Could you check a few things on this model? Use its own coordinates, in mm. A direction names the side the tool comes from. Give positions to 0.01 mm unless a question says otherwise; leave off trailing zeros. Order: outer loops, then holes, each group sorted by start corner. A loop starts at its lowest first (then second) coordinate and runs counter-clockwise, first axis right, second up. Notation, with made-up numbers: M 74.25,63 L 96.25,63 A21 cw 96.25,81 Z; hole C 72.25,51 d7. An arc over 180 degrees is marked long. Use a Markdown table: item, result. Add a question column.
Item 1: I'm going to push flat-ended pins straight in: pin 1 Ø1.2 at (x, y) = (-14, -3) entering from +Z; pin 2 Ø4.5 at (y, z) = (-2.5, 44) entering from -X; pin 3 Ø4 at (x, y) = (-9.5, 0) entering from +Z. Where does each tip first touch, or does it pass through?
Item 2: If we mould it in two halves opening along X, with no side actions, what happens to faces 4 (the face through (26.682, -1.485, 73.95)), 5 (the face through (-0.195, 2.972, 131.487)), 6 (the face through (0, 5, 76))? For each: released by +X, released by -X, zero draft, split by the parting line, or undercut.
Item 3: Suppose I cut it at A-A on x = 15. Write out the boundary of the cut face in (y, z).
Item 4: Suppose I cut it at B-B on z = 99. Write out the boundary of the cut face in (x, y).
Item 5: If I drill on L1, parallel to Z at x = -18, y = 1; L2, parallel to Z at x = 0, y = 3.55; L3, parallel to Z at x = 0, y = 2.15, over which ranges is the centre line in solid material (lowest first)? Write a range as from..to.
Item 6: For faces 1 (the face through (-0.42, -1.485, 3.318)), 2 (the face through (15, 1, 24)), 3 (the face through (19, 2, 48)), which set-ups out of +Z, -Z, +X, -X, +Y, -Y let a thin tool reach every point of the face, with its end or its side?
Item 7: Suppose I cut it at C-C on x = 0. Count the separate pieces of the cut face and the enclosed holes in it, plus the area to 3 significant figures.
from build123d import *
from build123d import SkipClean  # not in build123d's __all__

# Parameters (mm, degrees)
F0_R        = 1.5
F1_DEPTH    = 5
F0_W        = 22
F0_H        = 2
F0_W_2      = 2
F0_H_2      = 6
F0_W_3      = 4
F2_DEPTH    = 4
F3_SIZE     = 5
F4_T1_DEPTH = 109.7493718553
F4_T3_DEPTH = 199.7493718553


# Not quite as in the source:
# - a fillet or chamfer that OpenCascade refuses, or shapes differently, is made with other operations: its cross-section is extruded or revolved along the edge and cut away or added
# - a feature names something its author has since deleted; it is built from what else it names


with BuildPart() as f1:
    # F0 (on Front) → F1 (new body)
    with BuildSketch(Plane.XZ):
        with BuildLine():
            Line((-30, 150), (-30, 80))
            Line((-30, 80), (-1.5, 80))
            ThreePointArc((-1.5, 80), (0, 81.5), (1.5, 80))
            Line((1.5, 80), (30, 80))
            Line((30, 80), (30, 150))
            Line((30, 150), (-30, 150))
        make_face()
        with Locations((0, 130)):
            Circle(F0_R, mode=Mode.SUBTRACT)
        with BuildLine():
            Line((-30, 0), (0, 0))
            Line((0, 0), (30, 0))
            Line((30, 0), (30, 80))
            Line((30, 80), (1.5, 80))
            ThreePointArc((1.5, 80), (0, 78.5), (-1.5, 80))
            Line((-1.5, 80), (-30, 80))
            Line((-30, 80), (-30, 0))
        make_face()
        Polygon((-11, 24), (-11, 16), (-11, 10), (-11, 8), (-13, 8), (-17, 8), (-19, 8), (-19, 10), (-19, 16), (-19, 24), align=None, mode=Mode.SUBTRACT)
        Polygon((19, 24), (19, 16), (19, 10), (19, 8), (17, 8), (13, 8), (11, 8), (11, 10), (11, 16), (11, 24), align=None, mode=Mode.SUBTRACT)
        Polygon((-19, 54), (-11, 54), (11, 54), (19, 54), (19, 46), (19, 40), (19, 38), (17, 38), (13, 38), (11, 38), (-11, 38), (-13, 38), (-17, 38), (-19, 38), (-19, 40), (-19, 46), (-19, 48), align=None, mode=Mode.SUBTRACT)
    extrude(amount=-F1_DEPTH)

    # F0 (on Front) → F2 (join)
    with BuildSketch(Plane.XZ):
        with BuildLine():
            Line((-30, 0), (0, 0))
            Line((0, 0), (30, 0))
            Line((30, 0), (30, 80))
            Line((30, 80), (1.5, 80))
            ThreePointArc((1.5, 80), (0, 78.5), (-1.5, 80))
            Line((-1.5, 80), (-30, 80))
            Line((-30, 80), (-30, 0))
        make_face()
        Polygon((-11, 24), (-11, 16), (-11, 10), (-11, 8), (-13, 8), (-17, 8), (-19, 8), (-19, 10), (-19, 16), (-19, 24), align=None, mode=Mode.SUBTRACT)
        Polygon((19, 24), (19, 16), (19, 10), (19, 8), (17, 8), (13, 8), (11, 8), (11, 10), (11, 16), (11, 24), align=None, mode=Mode.SUBTRACT)
        Polygon((-19, 54), (-11, 54), (11, 54), (19, 54), (19, 46), (19, 40), (19, 38), (17, 38), (13, 38), (11, 38), (-11, 38), (-13, 38), (-17, 38), (-19, 38), (-19, 40), (-19, 46), (-19, 48), align=None, mode=Mode.SUBTRACT)
        with BuildLine():
            Line((-30, 150), (-30, 80))
            Line((-30, 80), (-1.5, 80))
            ThreePointArc((-1.5, 80), (0, 81.5), (1.5, 80))
            Line((1.5, 80), (30, 80))
            Line((30, 80), (30, 150))
            Line((30, 150), (-30, 150))
        make_face()
        with Locations((0, 130)):
            Circle(F0_R, mode=Mode.SUBTRACT)
        with Locations((0, 39)):
            Rectangle(F0_W, F0_H)
        with Locations((-18, 43)):
            Rectangle(F0_W_2, F0_H_2)
        with Locations((18, 43)):
            Rectangle(F0_W_2, F0_H_2)
        with Locations((-18, 13)):
            Rectangle(F0_W_2, F0_H_2)
        with Locations((-12, 13)):
            Rectangle(F0_W_2, F0_H_2)
        with Locations((12, 13)):
            Rectangle(F0_W_2, F0_H_2)
        with Locations((18, 13)):
            Rectangle(F0_W_2, F0_H_2)
        with Locations((-15, 39)):
            Rectangle(F0_W_3, F0_H)
        with Locations((15, 39)):
            Rectangle(F0_W_3, F0_H)
        with Locations((-15, 9)):
            Rectangle(F0_W_3, F0_H)
        with Locations((15, 9)):
            Rectangle(F0_W_3, F0_H)
        with Locations((-18, 39)):
            Rectangle(F0_W_2, F0_H)
        with Locations((-12, 39)):
            Rectangle(F0_W_2, F0_H)
        with Locations((12, 39)):
            Rectangle(F0_W_2, F0_H)
        with Locations((18, 39)):
            Rectangle(F0_W_2, F0_H)
        with Locations((-18, 9)):
            Rectangle(F0_W_2, F0_H)
        with Locations((-12, 9)):
            Rectangle(F0_W_2, F0_H)
        with Locations((12, 9)):
            Rectangle(F0_W_2, F0_H)
        with Locations((18, 9)):
            Rectangle(F0_W_2, F0_H)
    with SkipClean():  # cleaning this boolean's faces spoils the solid; the shape is the same uncleaned
        extrude(amount=F2_DEPTH)

    # F3
    f3_edges = [f1.edges().sort_by_distance(p)[0] for p in [
        (-1.5, -4, 130),
        (1.5, -4, 80),
    ]]
    chamfer(f3_edges, length=F3_SIZE)

    # F4: fillet of radius 10 on 4 edges, made by hand

    # F4_s2 → F4_t1 (cut)
    with BuildSketch(Plane.YZ.offset(-54.8746859277)):
        with BuildLine():
            ThreePointArc((-4, 9.9498743711), (-1.4161984871, 3.2416704386), (5, 0))
            Line((5, 0), (-4, 0))
            Line((-4, 0), (-4, 9.9498743711))
        make_face()
        with BuildLine():
            ThreePointArc((-4, 140.0501256289), (-1.4161984871, 146.7583295614), (5, 150))
            Line((5, 150), (-4, 150))
            Line((-4, 150), (-4, 140.0501256289))
        make_face()
    extrude(amount=F4_T1_DEPTH, mode=Mode.SUBTRACT)

    # F4_s4 → F4_t3 (cut)
    with BuildSketch(Plane.XY.offset(-24.8746859277)):
        with BuildLine():
            ThreePointArc((-20.0501256289, -4), (-26.7583295614, -1.4161984871), (-30, 5))
            Line((-30, 5), (-30, -4))
            Line((-30, -4), (-20.0501256289, -4))
        make_face()
        with BuildLine():
            ThreePointArc((20.0501256289, -4), (26.7583295614, -1.4161984871), (30, 5))
            Line((30, 5), (30, -4))
            Line((30, -4), (20.0501256289, -4))
        make_face()
    extrude(amount=F4_T3_DEPTH, mode=Mode.SUBTRACT)


solid = f1.part
Findings below:
| question | item | result |
|---|---|---|
| 1 | pin 1 | stops at z = 145.48 |
| 1 | pin 2 | stops at x = -27.86 |
| 1 | pin 3 | stops at z = 149.22 |
| 2 | face 4 | released by +X |
| 2 | face 5 | undercut |
| 2 | face 6 | zero draft |
| 3 | outline | M -4,9.95 A10 ccw 5,0 L 5,8 L 0,8 L 0,10 L -4,10 Z; M -4,24 L 5,24 L 5,38 L 0,38 L 0,40 L -4,40 Z; M -4,54 L 5,54 L 5,150 A10 ccw -4,140.05 Z |
| 4 | outline | M -30,5 A10 ccw -20.05,-4 L 20.05,-4 A10 ccw 30,5 Z |
| 5 | L1 | z = 1.29..8, 24..38, 54..148.71 |
| 5 | L2 | z = 0.25..38, 54..78.5, 81.5..128.5, 131.5..149.75 |
| 5 | L3 | z = 0.72..38, 54..78.5, 81.5..128.5, 131.5..149.28 |
| 6 | face 1 | -Z, +X, -X, -Y |
| 6 | face 2 | +Y, -Y |
| 6 | face 3 | +Y |
| 7 | separate pieces | 4 |
| 7 | enclosed holes | 0 |
| 7 | area | 1,070 mm^2 |
